For this review, take the finished solid that the model builds, in its own axes (mm). Coordinates: 2 decimals unless noted, no trailing zeros. Loops run counter-clockwise (first coordinate to the right, second up) from the corner with the lowest first, then second, coordinate; pieces in that order, holes last. Notation, with made-up numbers: M 79,11.25 L 98,11.25 A24 ccw 98,34.25 Z; hole C 51.25,7.5 d7. An arc over 180 degrees is marked long. Write each question's results on one line, items separated by ' | '. Start each with the question number.
```python
from build123d import *

# Parameters (mm, degrees)
F0_W     = 23.8125
F0_H     = 19.05
F1_DEPTH = 215.9
F3_DEPTH = 25.4
F5_D     = 6.35
F5_DEPTH = 50.8
F5_TIP   = 1.9077324654
F7_D     = 6.35
F7_DEPTH = 50.8
F7_TIP   = 1.9077324654


with BuildPart() as f1:
    # F0 (on Front) → F1 (new body)
    with BuildSketch(Plane.XZ):
        with Locations((11.90625, 9.525)):
            Rectangle(F0_W, F0_H)
    extrude(amount=F1_DEPTH)

    # F2 (on Right) → F3 (cut)
    with BuildSketch(Plane.YZ):
        Polygon((-125.693321228, 23.7295310944), (-152.0250290632, 23.7955264747), (-144.0397202969, 13.7644028291), (-131.6988021135, 13.7644028291), align=None)
        Polygon((-130.116969347, 34.1722927988), (-152.0250290632, 23.7955264747), (-125.693321228, 23.7295310944), align=None)
    extrude(amount=F3_DEPTH, mode=Mode.SUBTRACT)

    # F5
    with Locations(Plane(origin=(0, 0, 0), x_dir=(0, 1, 0), z_dir=(-1, 0, 0))):
        with Locations((-6.35, -12.2258998454)):
            Hole(F5_D / 2, depth=F5_DEPTH)
            with Locations((0, 0, -(F5_DEPTH + F5_TIP / 2))):  # 118° drill point
                Cone(0, F5_D / 2, F5_TIP, mode=Mode.SUBTRACT)

    # F7
    with Locations(Plane(origin=(0, 0, 0), x_dir=(0, 1, 0), z_dir=(-1, 0, 0))):
        with Locations((-209.7170012236, -11.3129783422)):
            Hole(F7_D / 2, depth=F7_DEPTH)
            with Locations((0, 0, -(F7_DEPTH + F7_TIP / 2))):  # 118° drill point
                Cone(0, F7_D / 2, F7_TIP, mode=Mode.SUBTRACT)


solid = f1.part
```
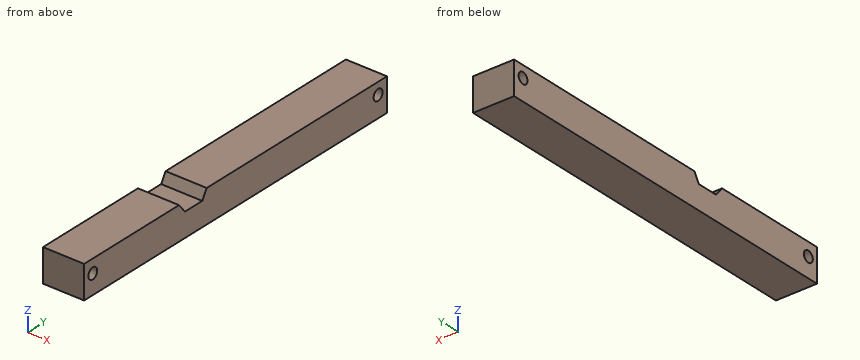
Q1. Insertion check: P1, Ø13.5, axis at x = 13, y = -138, coming from the +Z side; P2, Ø5.5, axis at y = -209.72, z = 11.31, coming from the +X side. Each pin has a flat end and moves straight along its axis. Give the tip position at first contact, or say it passes through.
Q2. Take a section at A-A, the plane y = -6.35. Give the boundary of the cut face in (x, z), then the cut area to 3 significant figures.
Q3. Take a section at B-B, the plane x = 6.75. Give the boundary of the cut face in (y, z) (3 decimals), then the cut area to 3 significant figures.
Q4. To check wall thickness, follow line 1 along Z through (x, y) = (5, -6.35); line 2 along Y through (x, z) = (6.75, 11); line 3 along Y through (x, z) = (20.5, 14.75). State the ranges of each line that lie inside material, in increasing order.
Results:
1) P1: z = 14.66 | P2: through
2) outline: M 0,0 L 23.81,0 L 23.81,9.05 L 0,9.05 Z; M 0,15.4 L 23.81,15.4 L 23.81,19.05 L 0,19.05 Z | area: 302 mm^2
3) outline: M -215.9,0 L 0,0 L 0,19.05 L -128.513,19.05 L -131.699,13.764 L -144.04,13.764 L -148.247,19.05 L -215.9,19.05 Z; hole C -209.717,11.313 d6.35; hole C -6.35,12.226 d6.35 | area: 3,960 mm^2
4) line 1: 0 to 9.05, 15.4 to 19.05 | line 2: -215.9 to -212.88, -206.56 to -9.28, -3.42 to 0 | line 3: -215.9 to -144.82, -131.1 to -8.28, -4.42 to 0
